```python
from build123d import *

# Parameters (mm, degrees)
PAD_DEPTH           = 6
HOLE_D              = 2.4
HOLE_CBORE_D        = 4.3
HOLE_CBORE_DEPTH    = 1.6
HOLE001_D           = 2.4
HOLE001_CBORE_D     = 4.3
HOLE001_CBORE_DEPTH = 1.6


with BuildPart() as part:
    # Sketch001 → Pad (new body)
    with BuildSketch(Plane(origin=(-8.845912, -9.712389, 7.5), x_dir=(1, 0, 0), z_dir=(0, 1, 0))):
        Polygon((3.85, 8.5), (-1.15, 14.5), (-4.15, 14.5), (-4.15, -14.5), (-1.15, -14.5), (3.85, -8.5), (6.85, -8.5), (-0.15, -17.5), (-0.15, -40), (40.85, -40), (48.85, -43), (50.85, -43), (50.85, -50), (-9.15, -50), (-9.15, -17.5), (-9.15, 17.5), (-9.15, 50), (50.85, 50), (50.85, 43), (48.85, 43), (40.85, 40), (-0.15, 40), (-0.15, 17.5), (6.85, 8.5), align=None)
    extrude(amount=PAD_DEPTH)

    # Hole (through all)
    with Locations(Plane(origin=(-8.845912, -9.712389, 7.5), x_dir=(1, 0, 0), z_dir=(0, -1, 0))):
        with Locations((-6.654088, 0), (-6.654088, 15), (-6.654088, -15)):
            CounterBoreHole(HOLE_D / 2, HOLE_CBORE_D / 2, HOLE_CBORE_DEPTH)

    # Hole001 (through all)
    with Locations(Plane(origin=(-8.845912, -9.712389, 7.5), x_dir=(1, 0, 0), z_dir=(0, -1, 0))):
        with Locations((20.595912, 44.973288), (20.595912, -45.026712), (-4.654088, -45.026712), (45.845912, -45.026712), (-4.654088, 44.973288), (45.845912, 44.973288)):
            CounterBoreHole(HOLE001_D / 2, HOLE001_CBORE_D / 2, HOLE001_CBORE_DEPTH)


solid = part.part
```
Source: CAD feature listing. Evaluate the final solid. Frame: model axes, mm. A direction names the side the tool comes from. Round coordinates to 2 decimals unless told otherwise and drop trailing zeros. Loops run counter-clockwise (first coordinate to the right, second up) from the corner with the lowest first, then second, coordinate; pieces in that order, holes last. Notation, with made-up numbers: M 6.5,53 L 52.5,53 A21 cw 52.5,69 Z; hole C 74,6 d7. An arc over 180 degrees is marked long. Use a Markdown table: item, result. Add a question column.
1. Mould query, pull axis Z, two halves, no side actions, for faces 1 (the flat face through (-14, -8.112, 23)), 2 (the flat face through (12, -7, -42.5)), 3 (the cylindrical face through (-14.34, -8.92, -5.69)). Classes: pulls with the +Z half, pulls with the -Z half, needs draft (parallel to the pull), parting line crosses it, or undercut.
2. Reachability of faces 4 (the flat face through (38.4, -8.112, 52.5)), 5 (the flat face through (-11, -7, -7)), 6 (the flat face through (-5.45, -6.75, 20.44)) from +Z, -Z, +X, -X, +Y, -Y: full face, straight path, thin tool, end or side. Return the list, or none.
3. Line query: line 1 (Z direction, x = -13.5, y = -5.75); line 2 (Z direction, x = 11, y = -4.7); line 3 (Z direction, x = 28, y = -7.2). Output: solid intervals per line, ascending.
4. Section query C-C on z = 7.5. Return the cut outline in (x, y).
5. Section query D-D on y = -5.95. Give the number of separate pieces and of enclosed holes in the cut face, then the cut area to 3 significant figures.
6. Section query B-B on x = 29.5. Return the cut outline in (y, z), then the cut area to 3 significant figures.
7. Contact query for flat-ended pins moving along their axis: P1, Ø3.5, axis at x = -16.5, z = -8.5, coming from the -Y side; P2, Ø1.9, axis at x = -15.5, z = 22.5, coming from the +Y side; P3, Ø1.3, axis at x = 12.5, z = 51.5, coming from the -Y side. Output: stop coordinate, or through.
8. Section query A-A on x = 11.75. Return the cut outline in (y, z).
Reported:
| question | item | result |
|---|---|---|
| 1 | face 1 | undercut |
| 1 | face 2 | pulls with the -Z half |
| 1 | face 3 | undercut |
| 2 | face 4 | -Y |
| 2 | face 5 | +Y, -Y |
| 2 | face 6 | +X, +Y, -Y |
| 3 | line 1 | z = -42.5 to -38.73, -36.33 to 51.27, 53.67 to 57.5 |
| 3 | line 2 | z = -42.5 to -38.46, -36.59 to -32.5, 47.5 to 51.54, 53.41 to 57.5 |
| 3 | line 3 | z = -42.5 to -32.5, 47.5 to 57.5 |
| 4 | outline | M -18,-9.71 L -17.65,-9.71 L -17.65,-8.11 L -16.7,-8.11 L -16.7,-3.71 L -18,-3.71 Z; M -14.3,-8.11 L -13.35,-8.11 L -13.35,-9.71 L -13,-9.71 L -13,-3.71 L -14.3,-3.71 Z |
| 5 | separate pieces | 1 |
| 5 | enclosed holes | 9 |
| 5 | area | 1,770 mm² |
| 6 | outline | M -9.71,-42.5 L -3.71,-42.5 L -3.71,-32.5 L -9.71,-32.5 Z; M -9.71,47.5 L -3.71,47.5 L -3.71,57.5 L -9.71,57.5 Z |
| 6 | area | 120 mm² |
| 7 | P1 | stops at y = -9.71 |
| 7 | P2 | passes through |
| 7 | P3 | stops at y = -8.11 |
| 8 | outline | M -9.71,-42.5 L -3.71,-42.5 L -3.71,-38.73 L -8.11,-38.73 L -8.11,-39.68 L -9.71,-39.68 Z; M -9.71,-35.38 L -8.11,-35.38 L -8.11,-36.33 L -3.71,-36.33 L -3.71,-32.5 L -9.71,-32.5 Z; M -9.71,47.5 L -3.71,47.5 L -3.71,51.27 L -8.11,51.27 L -8.11,50.32 L -9.71,50.32 Z; M -9.71,54.62 L -8.11,54.62 L -8.11,53.67 L -3.71,53.67 L -3.71,57.5 L -9.71,57.5 Z |
